Can you work these out from the model? Positions are in its coordinate system, mm. A direction names the side the tool comes from. Round coordinates to 2 decimals unless told otherwise and drop trailing zeros. Loops run counter-clockwise (first coordinate to the right, second up) from the corner with the lowest first, then second, coordinate; pieces in that order, holes last.
from build123d import *

# Parameters (mm, degrees)
SKETCH1_W                       = 25
SKETCH1_H                       = 4.9
BOSS_EXTRUDE1_DEPTH             = 30
SKETCH2_W                       = 9.9
SKETCH2_H                       = 4.9
BOSS_EXTRUDE2_DEPTH             = 10
CBORE_FOR_M3_SBHCS2_D           = 2.8
CBORE_FOR_M3_SBHCS2_CBORE_D     = 5.5
CBORE_FOR_M3_SBHCS2_CBORE_DEPTH = 3.1


with BuildPart() as part:
    # Sketch1 → Boss-Extrude1 (new, symmetric)
    with BuildSketch(Plane(origin=(0, 0, 0), x_dir=(0, 0, -1), z_dir=(1, 0, 0))):
        Rectangle(SKETCH1_W, SKETCH1_H)
    extrude(amount=BOSS_EXTRUDE1_DEPTH, both=True)

    # Sketch2 → Boss-Extrude2 (add)
    with BuildSketch(Plane(origin=(30, 0, 0), x_dir=(0, 0, -1), z_dir=(1, 0, 0))):
        Rectangle(SKETCH2_W, SKETCH2_H)
    boss_extrude2 = extrude(amount=BOSS_EXTRUDE2_DEPTH)

    # Mirror1: Boss-Extrude2 across plane
    add(boss_extrude2.mirror(Plane(origin=(0, 0, 0), x_dir=(0, 0, 1), z_dir=(1, 0, 0))))

    # CBORE for M3 SBHCS2 (through all)
    with Locations(Plane(origin=(0, -2.45, 0), x_dir=(-1, 0, 0), z_dir=(0, -1, 0))):
        with Locations((-8, 6), (8, 6), (8, -6), (-8, -6)):
            CounterBoreHole(CBORE_FOR_M3_SBHCS2_D / 2, CBORE_FOR_M3_SBHCS2_CBORE_D / 2, CBORE_FOR_M3_SBHCS2_CBORE_DEPTH)


solid = part.part
(1) Will these pins go through, and if not, where does the flat tip stop? P1, Ø2.5, axis at x = -34.5, y = 1, coming from the +Z side; P2, Ø1.5, axis at y = 1, z = -8, coming from the +X side; P3, Ø1.5, axis at x = -33, y = -0.5, coming from the -Z side.
Worked answers:
P1: stops at z = 4.95
P2: stops at x = 30
P3: stops at z = -4.95
(2) If we section it at A-A, the plane z = 6: List the corners of the cut face in (x, y) for me, then the cut area to 3 significant figures.
Worked answers:
outline: (-30, -2.45) - (-10.75, -2.45) - (-10.75, 0.65) - (-9.4, 0.65) - (-9.4, 2.45) - (-30, 2.45) - close; (-6.6, 0.65) - (-5.25, 0.65) - (-5.25, -2.45) - (5.25, -2.45) - (5.25, 0.65) - (6.6, 0.65) - (6.6, 2.45) - (-6.6, 2.45) - close; (9.4, 0.65) - (10.75, 0.65) - (10.75, -2.45) - (30, -2.45) - (30, 2.45) - (9.4, 2.45) - close
area: 250 mm2
(3) If I drill on line 1 (Z direction, x = 8, y = -0.3); line 2 (Z direction, x = -8, y = 1.7); line 3 (X direction, y = -1.75, z = 4.75), over which ranges is the centre line in solid material (lowest first)?
Worked answers:
line 1: z = -12.5 to -8.75, -3.25 to 3.25, 8.75 to 12.5
line 2: z = -12.5 to -7.4, -4.6 to 4.6, 7.4 to 12.5
line 3: x = -40 to -10.45, -5.55 to 5.55, 10.45 to 40
(4) For faces 1 (the flat face through (6.8, 0.65, -4.8)), 2 (the flat face through (40, 0, 0)), 3 (the flat face through (30, 0, 9)), 4 (the flat face through (-35, 0, -4.95)), 5 (the flat face through (-35, 0, 4.95)), which set-ups out of +Z, -Z, +X, -X, +Y, -Y let a thin tool reach every point of the face, with its end or its side?
Worked answers:
face 1: -Y
face 2: +Z, -Z, +X, +Y, -Y
face 3: +Z, +X, +Y, -Y
face 4: -Z, -X, +Y, -Y
face 5: +Z, -X, +Y, -Y
(5) If we section it at C-C, the plane y = -1.65: List the corners of the cut face in (x, z) for me.
Worked answers:
outline: (-40, -4.95) - (-30, -4.95) - (-30, -12.5) - (30, -12.5) - (30, -4.95) - (40, -4.95) - (40, 4.95) - (30, 4.95) - (30, 12.5) - (-30, 12.5) - (-30, 4.95) - (-40, 4.95) - close; hole circle Ø5.5 at (-8, -6); hole circle Ø5.5 at (-8, 6); hole circle Ø5.5 at (8, -6); hole circle Ø5.5 at (8, 6)
(6) If we mould it in two halves opening along X, with no side actions, what happens to faces 6 (the cylindrical face through (6.97, 1.56, -6.95)), 7 (the flat face through (-40, 0, 0)), 8 (the flat face through (35, 0, -4.95))? For each: released by +X, released by -X, zero draft, split by the parting line, or undercut.
Worked answers:
face 6: undercut
face 7: released by -X
face 8: zero draft
(7) If we section it at B-B, the plane x = 8: List the corners of the cut face in (y, z) for me.
Worked answers:
outline: (-2.45, -12.5) - (2.45, -12.5) - (2.45, -7.4) - (0.65, -7.4) - (0.65, -8.75) - (-2.45, -8.75) - close; (-2.45, -3.25) - (0.65, -3.25) - (0.65, -4.6) - (2.45, -4.6) - (2.45, 4.6) - (0.65, 4.6) - (0.65, 3.25) - (-2.45, 3.25) - close; (-2.45, 8.75) - (0.65, 8.75) - (0.65, 7.4) - (2.45, 7.4) - (2.45, 12.5) - (-2.45, 12.5) - close
